Part model, mm, in its own coordinate system. Face numbers are marked on the shaded views. A direction names the side the tool comes from. Give positions to 0.01 mm unless a question says otherwise; leave off trailing zeros. Write each loop counter-clockwise with the first axis right and the second up, starting at its lowest first coordinate (ties: lowest second). Pieces come first, ordered by that corner, then holes.
```python
from build123d import *

# Parameters (mm, degrees)
F1_DEPTH = 750
F2_R     = 2
F3_R     = 4
F4_R     = 19.05
F5_DEPTH = 15
F6_R     = 19.05
F7_DEPTH = 20


with BuildPart() as f1:
    # F0 (on Right) → F1 (new body, symmetric)
    with BuildSketch(Plane.YZ):
        Polygon((300, -75), (-300, -75), (-300, 75), (-302, 75), (-302, -77), (302, -77), (302, 75), (300, 75), align=None)
    extrude(amount=F1_DEPTH, both=True)

    # F2
    f2_edges = [f1.edges().sort_by_distance(p)[0] for p in [
        (0, 300, -75),
        (0, -300, -75),
    ]]
    fillet(f2_edges, radius=F2_R)

    # F3
    f3_edges = [f1.edges().sort_by_distance(p)[0] for p in [
        (0, -302, -77),
        (0, 302, -77),
    ]]
    fillet(f3_edges, radius=F3_R)

    # F4 (on face) → F5 (cut)
    with BuildSketch(Plane.XZ.offset(302)):
        with Locations((-720, -60)):
            Circle(F4_R)
        with Locations((-350, -60)):
            Circle(F4_R)
    extrude(amount=-F5_DEPTH, mode=Mode.SUBTRACT)

    # F6 (on face) → F7 (cut)
    with BuildSketch(Plane(origin=(-750, 0, 0), x_dir=(0, -1, 0), z_dir=(-1, 0, 0))):
        with Locations((70, -60)):
            Circle(F6_R)
    extrude(amount=-F7_DEPTH, mode=Mode.SUBTRACT)


solid = f1.part
```
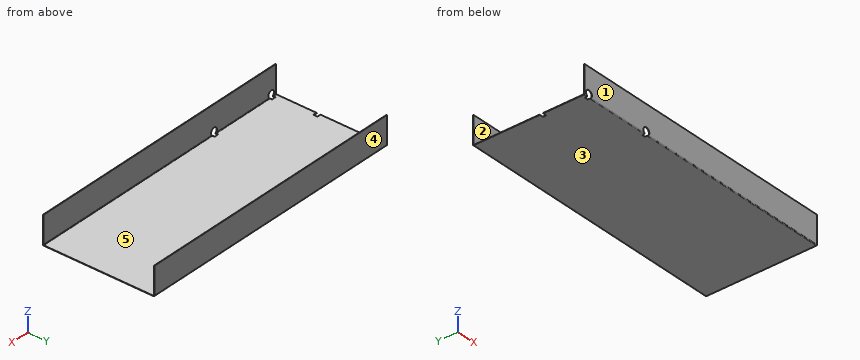
1) Saw through at C-C, the plane z = 30.5. Write the cut outline in (x, y).
Answers follow:
outline: (-750, -302) - (750, -302) - (750, -300) - (-750, -300) - close; (-750, 300) - (750, 300) - (750, 302) - (-750, 302) - close
2) Saw through at B-B, the plane x = -299. Write the cut outline in (y, z), then the cut area to 3 significant figures.
Answers follow:
outline: (-302, -73) arc R4 ccw to (-298, -77) - (298, -77) arc R4 ccw to (302, -73) - (302, 75) - (300, 75) - (300, -73) arc R2 cw to (298, -75) - (-298, -75) arc R2 cw to (-300, -73) - (-300, 75) - (-302, 75) - close
area: 1,800 mm2
3) Saw through at D-D, the plane y = 38. Write the cut outline in (x, z), then the cut area to 3 significant figures.
Answers follow:
outline: (-750, -77) - (750, -77) - (750, -75) - (-750, -75) - close
area: 3,000 mm2
4) Saw through at A-A, the plane z = -60. Write the cut outline in (x, y).
Answers follow:
outline: (-750, -302) - (-739.05, -302) - (-739.05, -300) - (-750, -300) - close; (-750, 300) - (750, 300) - (750, 302) - (-750, 302) - close; (-700.95, -302) - (-369.05, -302) - (-369.05, -300) - (-700.95, -300) - close; (-330.95, -302) - (750, -302) - (750, -300) - (-330.95, -300) - close
5) 3-axis set-ups, long thin cutter, end or side, ignore diameter. For the marked faces 1 and 2: which of +Z, -Z, +X, -X, +Y, -Y reach the whole face in a straight line?
Answers follow:
face 1: +Z, -Z, +X, -X, -Y
face 2: +Z, +X, -X
6) Wall check: L1, parallel to Y at x = -622, z = -4.5; L2, parallel to Z at x = 180.5, y = -80.5. Give the ranges that are in metal, low to high.
Answers follow:
L1: y = -302 to -300, 300 to 302
L2: z = -77 to -75
7) Two-plate mould, pull along Y, no slides. Class the marked faces 3, 4 and 5: +Y half, -Y half, draft (parallel to the pull), parting line (faces both ways), or undercut.
Answers follow:
face 3: draft
face 4: +Y half
face 5: undercut
8) Pin check, flat tips, straight feed: pin 1 Ø1.6 at (y, z) = (-66.5, -75.5) entering from -X; pin 2 Ø2 at (x, z) = (-719, -76) entering from -Y; pin 3 Ø12 at (x, y) = (-522.5, -132.5) entering from +Z. Stop position of each tip, or through.
Answers follow:
pin 1: stops at x = -730
pin 2: stops at y = -287
pin 3: stops at z = -75
